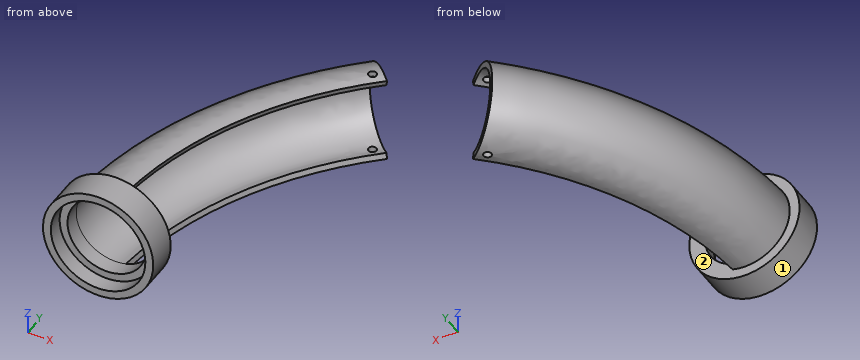
```python
from build123d import *

# Parameters (mm, degrees)
SKETCH2_R               = 88.9
SKETCH2_R_2             = 76.2
SKETCH2_R_3             = 63.5
BOSS_EXTRUDE1_DEPTH     = 50.8
SKETCH2_4_R             = 76.2
SKETCH2_4_R_2           = 63.5
CUT_EXTRUDE1_DEPTH      = 25.4
SKETCH5_R               = 6.35
CUT_EXTRUDE2_DEPTH      = 562.204013319
CUT_EXTRUDE2_DEPTH_BACK = 562.204013319


with BuildPart() as part:
    # Sketch2 → Boss-Extrude1 (new body)
    with BuildSketch(Plane(origin=(0, 0, 0), x_dir=(1, 0, 0), z_dir=(0, 1, 0))):
        with Locations(Location((0, 0, 0), (0, 0, 270))):
            Circle(SKETCH2_R)
        Circle(SKETCH2_R_2, mode=Mode.SUBTRACT)
        Circle(SKETCH2_R_2)
        with Locations(Location((0, 0, 0), (0, 0, 270))):
            Circle(SKETCH2_R_3, mode=Mode.SUBTRACT)
    extrude(amount=BOSS_EXTRUDE1_DEPTH)

    # Sketch2_4 → Cut-Extrude1 (cut)
    with BuildSketch(Plane(origin=(0, 0, 0), x_dir=(1, 0, 0), z_dir=(0, 1, 0))):
        with Locations(Location((0, 0, 0), (0, 0, 270))):
            Circle(SKETCH2_4_R)
        with Locations(Location((0, 0, 0), (0, 0, 270))):
            Circle(SKETCH2_4_R_2, mode=Mode.SUBTRACT)
    extrude(amount=CUT_EXTRUDE1_DEPTH, mode=Mode.SUBTRACT)

    # Sweep1: sweep along a path in Sketch3
    with BuildLine(Plane.XY) as sweep1_path:
        ThreePointArc((2.12035425, 50.8), (64.93047334, 273.764984481), (206.387500194, 457.2))
    # Sketch4 → Sweep1 (sweep)
    with BuildSketch(Plane(origin=(0, 50.8, 0), x_dir=(1, 0, 0), z_dir=(0, 1, 0))):
        with BuildLine():
            Line((16.435009364, 61.336289969), (18.900260769, 70.536733465))
            ThreePointArc((18.900260769, 70.536733465), (-73.025, 0), (18.900260769, -70.536733465))
            Line((18.900260769, -70.536733465), (16.435009364, -61.336289969))
            ThreePointArc((16.435009364, -61.336289969), (-63.5, 0), (16.435009364, 61.336289969))
        make_face()
    sweep(path=sweep1_path.line)

    # Sketch5 → Cut-Extrude2 (cut, two sides)
    with BuildSketch(Plane.XY) as cut_extrude2_sk:
        with Locations((194.61898253, 446.545535349)):
            Circle(SKETCH5_R)
    extrude(amount=CUT_EXTRUDE2_DEPTH, mode=Mode.SUBTRACT)
    extrude(cut_extrude2_sk.sketch, amount=-CUT_EXTRUDE2_DEPTH_BACK, mode=Mode.SUBTRACT)


solid = part.part
```
Geometry: final body of the model. Coordinates: model frame, mm. Face numbers are marked on the shaded views. Coordinates: 2 decimals unless noted, no trailing zeros. Return JSON: item names as keys, results as strings. Group by question number.
1. Pull-direction query (Y, two-part tool) for the marked faces 1 and 2; classes: pulls with the +Y half, pulls with the -Y half, needs draft (parallel to the pull), parting line crosses it, or undercut.
2. Pin query (flat end, axial travel): pin 1 (6 mm diameter, centred on y = 232, z = 42.5, fed in from +X); pin 2 (6 mm diameter, centred on x = 122, z = -6, fed in from -Y); pin 3 (3 mm diameter, centred on y = 260.5, z = 1, fed in from +X). Return the tip coordinate at first contact, or that it passes through.
3. Material intervals for line 1 along X through (y, z) = (32.75, 0); line 2 along X through (y, z) = (13.5, 0); line 3 along Z through (x, y) = (26, 170.5), sorted ascending. Write a range as [from, to].
Resolved:
{
 "1": {"face 1": "needs draft", "face 2": "undercut"},
 "2": {"pin 1": "stops at x = -3.67", "pin 2": "stops at y = 463.19", "pin 3": "stops at x = -12.48"},
 "3": {"line 1": "x = [-88.9, -63.5], [63.5, 88.9]", "line 2": "x = [-88.9, -76.2], [76.2, 88.9]", "line 3": "z = [-72.93, -63.39], [63.39, 72.93]"}
}
